Design review of the part built by this model. Coordinates are the model's own, in mm. Face numbers are marked on the shaded views. A direction names the side the tool comes from. Coordinates: 2 decimals unless noted, no trailing zeros. Order: outer loops, then holes, each group sorted by start corner. A loop starts at its lowest first (then second) coordinate and runs counter-clockwise, first axis right, second up.
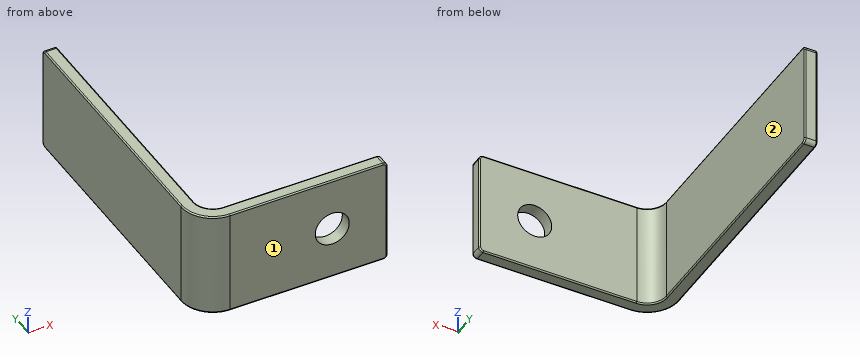
Autodesk Inventor part; units mm, degrees
ref_plane "YZ Plane" through (0, 0, 0) normal (1, 0, 0) x (0, 1, 0)
ref_plane "XZ Plane" through (0, 0, 0) normal (0, 1, 0) x (-1, 0, 0)
ref_plane "XY Plane" through (0, 0, 0) normal (0, 0, 1) x (1, 0, 0)
sketch "Sketch1" plane through (0, 0, 0) normal (0, 0, 1) x (1, 0, 0)
  line L0 (0, 0) -> (-37, 0)
  line L1 (-43, 6) -> (-43, 66)
  arc A0 (-43, 6) -> (-37, 0) centre (-37, 6) ccw
  point P0 (-43, 0)
  dimension "d0" = 43
  dimension "d1" = 66
  dimension "d2" = 6
sketch "Sketch2" plane through (0, 0, 0) normal (1, 0, 0) x (0, 1, 0)
  line L0 (-1.5, -12.5) -> (1.5, -12.5)
  line L1 (1.5, -12.5) -> (1.5, 12.5)
  line L2 (1.5, 12.5) -> (-1.5, 12.5)
  line L3 (-1.5, 12.5) -> (-1.5, -12.5)
  line L4 (-1.5, -12.5) -> (1.5, 12.5) construction
  line L5 (1.5, -12.5) -> (-1.5, 12.5) construction
  point P0 (0, 0)
  dimension "d3" = 3
  dimension "d4" = 25
sweep "Sweep1" add profiles "Sketch2" path "Sketch1"
sketch "Sketch3" plane through (0, 1.5, 12.5) normal (0, 1, 0) x (1, 0, 0)
  circle A0 centre (-13, 12.5) radius 4
  line L0 (0, 25) -> (0, 0)
  point P0 (0, 12.5)
  point P1 (0, 12.5)
  point P2 (0, 12.5)
  dimension "d7" = 8
  dimension "d8" = 13
extrude "Extrusion1" cut sketch "Sketch3" against normal through all
thread "Thread1"
fillet "Fillet1" radius 1 4 edges at (-43, 66, 12.5) (0, 0, 12.5) (0, 0, -12.5) (-43, 66, -12.5)
fillet "Fillet2" radius 0.3 24 edges at (-44.5, 65.7071, 12.2071) (-44.5, 66, 0) (-44.5, 65.7071, -12.2071) (-19, -1.5, -12.5) (-42.3033, 0.6967, -12.5) (-44.5, 35.5, -12.5) (-0.2929, -1.5, -12.2071) (0, -1.5, 0) (-0.2929, -1.5, 12.2071) (-19, -1.5, 12.5) (-42.3033, 0.6967, 12.5) (-44.5, 35.5, 12.5) (-41.5, 65.7071, 12.2071) (-41.5, 66, 0) (-41.5, 65.7071, -12.2071) (-19, 1.5, -12.5) (-40.182, 2.818, -12.5) (-41.5, 35.5, -12.5) (-0.2929, 1.5, -12.2071) (0, 1.5, 0) (-0.2929, 1.5, 12.2071) (-19, 1.5, 12.5) (-40.182, 2.818, 12.5) (-41.5, 35.5, 12.5)
properties part number "clampBaseBottom" material "Steel"
1. Add section D-D (z = -6.75). Give the boundary of the cut face in (x, y).
2. For the marked faces 1 and 2, list the 3-axis set-ups (+Z, -Z, +X, -X, +Y, -Y) from which the entire face can be reached by the end or side of a thin tool; tool diameter is ignored.
3. Add section A-A (z = 0). Give the boundary of the cut face in (x, y).
4. Add section C-C (y = 18). Give the boundary of the cut face in (x, z), and give its area (3 significant figures).
5. Add section B-B (x = -13). Give the boundary of the cut face in (y, z).
6. To check wall thickness, follow line 1 (Z direction, x = -13, y = -0.6); line 2 (X direction, y = 33.5, z = -3.5); line 3 (Y direction, x = -25.5, z = -10.75). State the ranges of each line that lie inside material, in increasing order.
7. Insertion check: pin 1 (5 mm diameter, centred on y = 56.5, z = 6.5, fed in from +X); pin 2 (2 mm diameter, centred on x = -8.5, z = -6.5, fed in from +Y). Each pin has a flat end and moves straight along its axis. Give the tip position at first contact, or say it passes through.
Solution:
1. outline: (-44.5, 6) arc R7.5 ccw to (-37, -1.5) - (-0.3, -1.5) arc R0.3 ccw to (0, -1.2) - (0, 1.2) arc R0.3 ccw to (-0.3, 1.5) - (-37, 1.5) arc R4.5 cw to (-41.5, 6) - (-41.5, 65.7) arc R0.3 ccw to (-41.8, 66) - (-44.2, 66) arc R0.3 ccw to (-44.5, 65.7) - close
2. face 1: +Z, -Z, +X, -X, -Y
2. face 2: +Z, -Z, +X, +Y
3. outline: (-44.5, 6) arc R7.5 ccw to (-37, -1.5) - (-17, -1.5) - (-17, 1.5) - (-37, 1.5) arc R4.5 cw to (-41.5, 6) - (-41.5, 65.7) arc R0.3 ccw to (-41.8, 66) - (-44.2, 66) arc R0.3 ccw to (-44.5, 65.7) - close; (-9, -1.5) - (-0.3, -1.5) arc R0.3 ccw to (0, -1.2) - (0, 1.2) arc R0.3 ccw to (-0.3, 1.5) - (-9, 1.5) - close
4. outline: (-44.5, -12.2) arc R0.3 ccw to (-44.2, -12.5) - (-41.8, -12.5) arc R0.3 ccw to (-41.5, -12.2) - (-41.5, 12.2) arc R0.3 ccw to (-41.8, 12.5) - (-44.2, 12.5) arc R0.3 ccw to (-44.5, 12.2) - close
4. area: 74.9 mm2
5. outline: (-1.5, -12.2) arc R0.3 ccw to (-1.2, -12.5) - (1.2, -12.5) arc R0.3 ccw to (1.5, -12.2) - (1.5, -4) - (-1.5, -4) - close; (-1.5, 4) - (1.5, 4) - (1.5, 12.2) arc R0.3 ccw to (1.2, 12.5) - (-1.2, 12.5) arc R0.3 ccw to (-1.5, 12.2) - close
6. line 1: z = -12.5 to -4, 4 to 12.5
6. line 2: x = -44.5 to -41.5
6. line 3: y = -1.5 to 1.5
7. pin 1: stops at x = -41.5
7. pin 2: stops at y = 1.5
